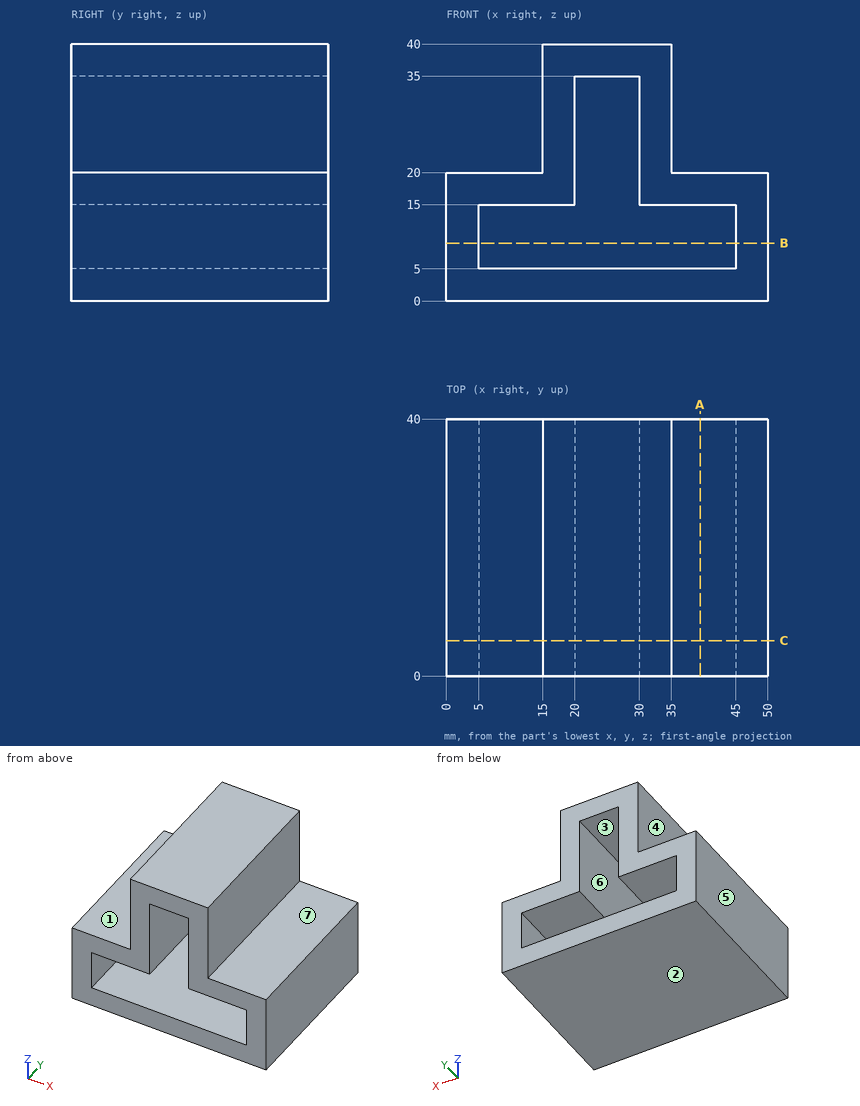
Check sheet for the drawn part. Datum: minimum x, y, z corner. Units: mm. A direction names the side the tool comes from. Round coordinates to 2 decimals unless told otherwise and drop trailing zeros. Loops run counter-clockwise (first coordinate to the right, second up) from the corner with the lowest first, then second, coordinate; pieces in that order, holes last. Notation, with made-up numbers: (-16.75, 34) - (38.25, 34) arc R11 ccw to (38.25, 48) - close; hole circle Ø3 at (-19.5, 56.25). An arc over 180 degrees is marked (long way). Use one line per item in the form item = value.
1. Section check B-B on z = 9. Record the cut outline in (x, y), and give its area (3 significant figures).
A:
outline = (0, 0) - (5, 0) - (5, 40) - (0, 40) - close; (45, 0) - (50, 0) - (50, 40) - (45, 40) - close
area = 400 mm²
2. Section check A-A on x = 39.5. Record the cut outline in (y, z), and give its area (3 significant figures).
A:
outline = (0, 0) - (40, 0) - (40, 5) - (0, 5) - close; (0, 15) - (40, 15) - (40, 20) - (0, 20) - close
area = 400 mm²
3. Access from +Z, -Z, +X, -X, +Y, -Y to the whole of each face (thin tool, end or side, straight path). Record for the marked faces 5, 6 and 7.
A:
face_5 = +Z, -Z, -X, +Y, -Y
face_6 = +Y, -Y
face_7 = +Z, +X, +Y, -Y
4. Draft check along Z on the marked faces 1, 2, 3 and 4. Enter one of: pulls with the +Z half, pulls with the -Z half, needs draft (parallel to the pull), parting line crosses it, or undercut.
A:
face_1 = pulls with the +Z half
face_2 = pulls with the -Z half
face_3 = undercut
face_4 = needs draft
5. Scan lines: probe 1 along Z at (x, y) = (22, 35); probe 2 along X at (y, z) = (28, 34); probe 3 along Z at (x, y) = (42, 21.5). Record each from-to range of solid material in increasing order.
A:
probe_1 = 0 to 5, 35 to 40
probe_2 = 15 to 20, 30 to 35
probe_3 = 0 to 5, 15 to 20
6. Section check C-C on y = 5.5. Record the cut outline in (x, z).
A:
outline = (0, 0) - (50, 0) - (50, 20) - (35, 20) - (35, 40) - (15, 40) - (15, 20) - (0, 20) - close; hole (5, 5) - (45, 5) - (45, 15) - (30, 15) - (30, 35) - (20, 35) - (20, 15) - (5, 15) - close
7. Gauge pin test, flat ends, axial feed: pin 1 Ø1 at (y, z) = (5.5, 28) entering from -X; pin 2 Ø5 at (y, z) = (20, 28.5) entering from +X; pin 3 Ø7.5 at (x, y) = (7, 19) entering from +Z. Record the tip position at first contact, or that the pin passes through.
A:
pin_1 = 15
pin_2 = 35
pin_3 = 20
